For this review, use the dimensioned drawing (mm, ordinates from the lowest corner) and the shaded views. A direction names the side the tool comes from. Round coordinates to 2 decimals unless told otherwise and drop trailing zeros. Loops run counter-clockwise (first coordinate to the right, second up) from the corner with the lowest first, then second, coordinate; pieces in that order, holes last. Notation, with made-up numbers: M -27.5,1 L -7.5,1 A16 cw -7.5,25 Z; hole C -27.5,-35.75 d2. An arc over 180 degrees is marked long. Use a Markdown table: item, result. Add a question column.
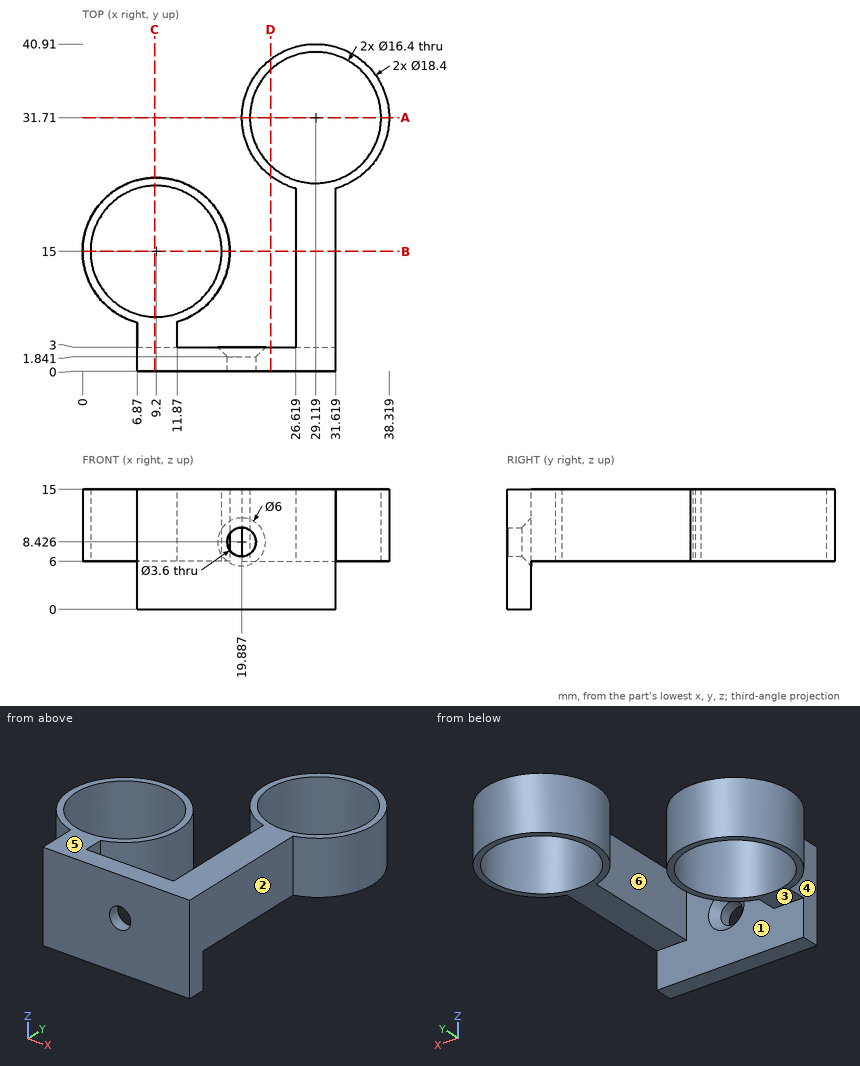
(1) Consider section D-D, the plane x = 23.5. Give the boundary of the cut face in (y, z) (1 decimal).
(2) Insertion check: pin 1 Ø6 at (x, z) = (6, 11.5) entering from +Y; pin 2 Ø1 at (y, z) = (31, 6) entering from -X; pin 3 Ø4.5 at (x, z) = (13.5, 6.5) entering from +Y; pin 4 Ø13 at (x, y) = (9.2, 15) entering from +Z. Each pin has a flat end and moves straight along its axis. Give the tip position at first contact, or say it passes through.
(3) Consider section C-C, the plane x = 9. Give the boundary of the cut face in (y, z).
(4) To check wall thickness, follow probe 1 along Y at (x, z) = (9.2, 10.25); probe 2 along Y at (x, z) = (12, 11.5); probe 3 along Y at (x, z) = (23.5, 9.75) (1 decimal). State the ranges of each line that lie inside material, in increasing order.
(5) For the marked faces 1, 2 and 3, list the 3-axis set-ups (+Z, -Z, +X, -X, +Y, -Y) from which the entire face can be reached by the end or side of a thin tool; tool diameter is ignored.
(6) Consider section B-B, the plane y = 15. Give the boundary of the cut face in (x, z), then the cut area to 3 significant figures.
(7) Draft analysis for pull direction X (two halves, no side actions). For the marked faces 4, 5 and 6, state which applies: released by +X, released by -X, zero draft, split by the parting line, or undercut.
(8) Consider section A-A, the plane y = 31.71. Give the boundary of the cut face in (x, z).
Found:
| question | item | result |
|---|---|---|
| 1 | outline | M 0,0 L 3,0 L 3,15 L 0,15 Z; M 24.4,6 L 25.7,6 L 25.7,15 L 24.4,15 Z; M 37.7,6 L 39,6 L 39,15 L 37.7,15 Z |
| 2 | pin 1 | stops at y = 24.2 |
| 2 | pin 2 | stops at x = 19.92 |
| 2 | pin 3 | stops at y = 23.97 |
| 2 | pin 4 | passes through |
| 3 | outline | M 0,0 L 3,0 L 3,6 L 6.8,6 L 6.8,15 L 0,15 Z; M 23.2,6 L 24.2,6 L 24.2,15 L 23.2,15 Z |
| 4 | probe 1 | y = 0 to 6.8, 23.2 to 24.2 |
| 4 | probe 2 | y = 0 to 3, 6.24 to 7.29, 22.71 to 23.76 |
| 4 | probe 3 | y = 0 to 3, 24.4 to 25.7, 37.7 to 39 |
| 5 | face 1 | -Z |
| 5 | face 2 | +Z, -Z, +X, -Y |
| 5 | face 3 | -Z, +X, -X, +Y |
| 6 | outline | M 0,6 L 1,6 L 1,15 L 0,15 Z; M 17.4,6 L 18.4,6 L 18.4,15 L 17.4,15 Z; M 26.62,6 L 31.62,6 L 31.62,15 L 26.62,15 Z |
| 6 | area | 63.0 mm^2 |
| 7 | face 4 | released by -X |
| 7 | face 5 | zero draft |
| 7 | face 6 | undercut |
| 8 | outline | M 19.92,6 L 20.92,6 L 20.92,15 L 19.92,15 Z; M 37.32,6 L 38.32,6 L 38.32,15 L 37.32,15 Z |
